Verification items for the finished model (mm, model axes). Face numbers are marked on the shaded views. Round coordinates to 2 decimals unless told otherwise and drop trailing zeros. Order: outer loops, then holes, each group sorted by start corner. A loop starts at its lowest first (then second) coordinate and runs counter-clockwise, first axis right, second up. Notation, with made-up numbers: M 86.5,4 L 120.5,4 A21 cw 120.5,9 Z; hole C -10,-39.5 d8. An arc over 180 degrees is marked long. Use one line per item in the form item = value. Start each with the question number.
Item 1: Cross-section at D-D on z = -85.5. Enter the section's corners in (x, y), then the cut area to 3 significant figures.
Item 2: Release check for a two-part mould opening along Z. For the marked faces 1 and 2 record: +Z half, -Z half, draft (parallel to the pull), parting line (faces both ways), or undercut.
Item 3: Cross-section at B-B on x = 52. Enter the section's corners in (y, z).
Item 4: Go/stop test with flat-tipped pins: pin 1 Ø2 at (x, z) = (68, -31.5) entering from -Y; pin 2 Ø12 at (x, z) = (65.5, -70.5) entering from +Y; pin 3 Ø8 at (x, z) = (42, -114) entering from -Y. Record where each tip stops, or that it passes through.
Item 5: Cross-section at A-A on x = 73. Enter the section's corners in (y, z), then the cut area to 3 significant figures.
Item 6: Cross-section at C-C on z = -99.5. Enter the section's corners in (x, y), then the cut area to 3 significant figures.
Item 7: Thickness scan on probe 1 along X at (y, z) = (-2, -29); probe 2 along Z at (x, y) = (38, 1.75); probe 3 along Z at (x, y) = (45, 4.75). Record the ranges inside material, lowest first. Write a range as [from, to].
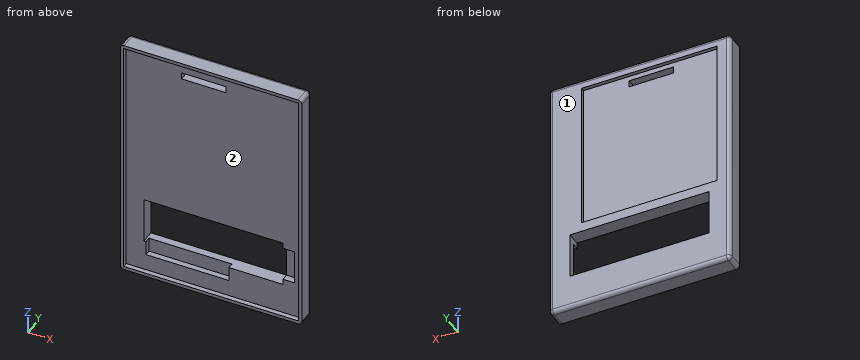
from build123d import *

# Parameters (mm, degrees)
SKETCH1_W           = 94
SKETCH1_H           = 130
BOSS_EXTRUDE1_DEPTH = 7
SKETCH2_W           = 72
SKETCH2_H           = 24
CUT_EXTRUDE1_DEPTH  = 8
SKETCH3_W           = 6
SKETCH3_H           = 18
CUT_EXTRUDE2_DEPTH  = 3.5
SKETCH4_W           = 43
SKETCH4_H           = 7.5
CUT_EXTRUDE3_DEPTH  = 3
SKETCH5_W           = 70
SKETCH5_H           = 78
CUT_EXTRUDE4_DEPTH  = 2
SKETCH6_W           = 23
SKETCH6_H           = 3.5
CUT_EXTRUDE5_DEPTH  = 6
FILLET1_R           = 2
SKETCH8_W           = 90.5
SKETCH8_H           = 126.5
BOSS_EXTRUDE2_DEPTH = 2.5


with BuildPart() as part:
    # Sketch1 → Boss-Extrude1 (new body)
    with BuildSketch(Plane(origin=(0, 0, 0), x_dir=(1, 0, 0), z_dir=(0, 1, 0))):
        with Locations((47, 65)):
            Rectangle(SKETCH1_W, SKETCH1_H)
    extrude(amount=BOSS_EXTRUDE1_DEPTH)

    # Sketch2 → Cut-Extrude1 (cut, through all)
    with BuildSketch(Plane(origin=(0, 7, 0), x_dir=(1, 0, 0), z_dir=(0, 1, 0))):
        with Locations((47, 100)):
            Rectangle(SKETCH2_W, SKETCH2_H)
    extrude(amount=-CUT_EXTRUDE1_DEPTH, mode=Mode.SUBTRACT)

    # Sketch3 → Cut-Extrude2 (cut)
    with BuildSketch(Plane.XZ):
        with Locations((86, -100)):
            Rectangle(SKETCH3_W, SKETCH3_H)
    extrude(amount=-CUT_EXTRUDE2_DEPTH, mode=Mode.SUBTRACT)

    # Sketch4 → Cut-Extrude3 (cut)
    with BuildSketch(Plane.XZ):
        with Locations((33.5, -115.75)):
            Rectangle(SKETCH4_W, SKETCH4_H)
    extrude(amount=-CUT_EXTRUDE3_DEPTH, mode=Mode.SUBTRACT)

    # Sketch5 → Cut-Extrude4 (cut)
    with BuildSketch(Plane(origin=(0, 7, 0), x_dir=(1, 0, 0), z_dir=(0, 1, 0))):
        with Locations((42, 44)):
            Rectangle(SKETCH5_W, SKETCH5_H)
    extrude(amount=-CUT_EXTRUDE4_DEPTH, mode=Mode.SUBTRACT)

    # Sketch6 → Cut-Extrude5 (cut, through all)
    with BuildSketch(Plane(origin=(0, 5, 0), x_dir=(1, 0, 0), z_dir=(0, 1, 0))):
        with Locations((42, 9.25)):
            Rectangle(SKETCH6_W, SKETCH6_H)
    extrude(amount=-CUT_EXTRUDE5_DEPTH, mode=Mode.SUBTRACT)

    # Fillet1
    fillet1_edges = [part.edges().sort_by_distance(p)[0] for p in [
        (94, 7, -65),
        (47, 7, -130),
        (0, 7, -65),
        (0, 3.5, -130),
        (94, 3.5, -130),
        (94, 3.5, 0),
        (0, 3.5, 0),
        (47, 7, 0),
    ]]
    fillet(fillet1_edges, radius=FILLET1_R)

    # Sketch8 → Boss-Extrude2 (add)
    with BuildSketch(Plane.XZ):
        with BuildLine():
            Line((92, -130), (2, -130))
            ThreePointArc((2, -130), (0.585786438, -129.414213562), (0, -128))
            Line((0, -128), (0, -2))
            ThreePointArc((0, -2), (0.585786438, -0.585786438), (2, 0))
            Line((2, 0), (92, 0))
            ThreePointArc((92, 0), (93.414213562, -0.585786438), (94, -2))
            Line((94, -2), (94, -128))
            ThreePointArc((94, -128), (93.414213562, -129.414213562), (92, -130))
        make_face()
        with Locations((47, -65)):
            Rectangle(SKETCH8_W, SKETCH8_H, mode=Mode.SUBTRACT)
    extrude(amount=BOSS_EXTRUDE2_DEPTH)


solid = part.part
Output values:
q1.outline = M 0,-2.5 L 1.75,-2.5 L 1.75,0 L 92.25,0 L 92.25,-2.5 L 94,-2.5 L 94,5 A2 ccw 92,7 L 2,7 A2 ccw 0,5 Z
q1.area = 665 mm2
q2.face_1 = draft
q2.face_2 = undercut
q3.outline = M -2.5,-130 L 5,-130 A2 ccw 7,-128 L 7,-112 L 3,-112 L 3,-119.5 L 0,-119.5 L 0,-128.25 L -2.5,-128.25 Z; M -2.5,-1.75 L 0,-1.75 L 0,-7.5 L 5,-7.5 L 5,-5 L 7,-5 L 7,-2 A2 ccw 5,0 L -2.5,0 Z; M 0,-88 L 7,-88 L 7,-83 L 5,-83 L 5,-11 L 0,-11 Z
q4.pin_1 = 0
q4.pin_2 = 5
q4.pin_3 = 3
q5.outline = M -2.5,-130 L 5,-130 A2 ccw 7,-128 L 7,-112 L 0,-112 L 0,-128.25 L -2.5,-128.25 Z; M -2.5,-1.75 L 0,-1.75 L 0,-88 L 7,-88 L 7,-83 L 5,-83 L 5,-5 L 7,-5 L 7,-2 A2 ccw 5,0 L -2.5,0 Z
q5.area = 593 mm2
q6.outline = M 0,-2.5 L 1.75,-2.5 L 1.75,0 L 11,0 L 11,7 L 2,7 A2 ccw 0,5 Z; M 83,3.5 L 89,3.5 L 89,0 L 92.25,0 L 92.25,-2.5 L 94,-2.5 L 94,5 A2 ccw 92,7 L 83,7 Z
q6.area = 140 mm2
q7.probe_1 = [0, 1.75], [92.25, 94]
q7.probe_2 = [-130, -119.5], [-88, -11], [-7.5, 0]
q7.probe_3 = [-130, -112], [-88, -11], [-7.5, 0]
